from build123d import *

# Parameters (mm, degrees)
BOSS_EXTRUDE3_DEPTH       = 17
SHELL4_T                  = -2.25
SHELL4_THICKNESS_2_FACE_W = 17.75
SHELL4_THICKNESS_2_FACE_H = 12.5
SHELL4_THICKNESS_2_DEPTH  = 0.75
SHELL4_THICKNESS_3_FACE_W = 17
SHELL4_THICKNESS_3_FACE_H = 12.5
SHELL4_THICKNESS_3_DEPTH  = 0.75
CUT_EXTRUDE1_DEPTH        = 29.08914381
CUT_EXTRUDE2_DEPTH        = 29.08914381
BOSS_EXTRUDE4_DEPTH       = 1
BOSS_EXTRUDE5_DEPTH       = 1
BOSS_EXTRUDE6_DEPTH       = 1
BOSS_EXTRUDE7_DEPTH       = 1


with BuildPart() as part:
    # Sketch4 → Boss-Extrude3 (new body)
    with BuildSketch(Plane(origin=(0, 0, 0), x_dir=(0, 0, -1), z_dir=(1, 0, 0))):
        Polygon((7, 10), (-10, -7), (-10, -10), (10, -10), (10, 10), align=None)
    extrude(amount=BOSS_EXTRUDE3_DEPTH)

    # Shell4
    shell4_openings = [part.faces().sort_by_distance(p)[0] for p in [
        (8.5, 10, -8.5),
        (8.5, -8.5, 10),
        (8.5, 1.5, 1.5),
    ]]
    offset(amount=SHELL4_T, openings=shell4_openings, kind=Kind.INTERSECTION)

    # Shell4 thickness 2 face (on inner face of the shell) → Shell4 thickness 2 (add)
    with BuildSketch(Plane(origin=(8.5, -7.75, 1.125), x_dir=(0, 0, -1), z_dir=(0, -1, 0))):
        Rectangle(SHELL4_THICKNESS_2_FACE_W, SHELL4_THICKNESS_2_FACE_H)
    extrude(amount=-SHELL4_THICKNESS_2_DEPTH)

    # Shell4 thickness 3 face (on inner face of the shell) → Shell4 thickness 3 (add)
    with BuildSketch(Plane(origin=(8.5, 1.5, -7.75), x_dir=(0, -1, 0), z_dir=(0, 0, -1))):
        Rectangle(SHELL4_THICKNESS_3_FACE_W, SHELL4_THICKNESS_3_FACE_H)
    extrude(amount=-SHELL4_THICKNESS_3_DEPTH)

    # Sketch5 → Cut-Extrude1 (cut, through all)
    with BuildSketch(Plane(origin=(0, 0, -10), x_dir=(-1, 0, 0), z_dir=(0, 0, -1))):
        with BuildLine():
            Line((-11.5, 1.5), (-11.5, -1.5))
            ThreePointArc((-11.5, -1.5), (-8.5, -4.5), (-5.5, -1.5))
            Line((-5.5, -1.5), (-5.5, 1.5))
            ThreePointArc((-5.5, 1.5), (-8.5, 4.5), (-11.5, 1.5))
        make_face()
    extrude(amount=-CUT_EXTRUDE1_DEPTH, mode=Mode.SUBTRACT)

    # Sketch8 → Cut-Extrude2 (cut, through all)
    with BuildSketch(Plane(origin=(0, -10, 0), x_dir=(-1, 0, 0), z_dir=(0, -1, 0))):
        with BuildLine():
            Line((-11.5, 1.5), (-11.5, -1.5))
            ThreePointArc((-11.5, -1.5), (-8.5, -4.5), (-5.5, -1.5))
            Line((-5.5, -1.5), (-5.5, 1.5))
            ThreePointArc((-5.5, 1.5), (-8.5, 4.5), (-11.5, 1.5))
        make_face()
    extrude(amount=-CUT_EXTRUDE2_DEPTH, mode=Mode.SUBTRACT)

    # Sketch9 → Boss-Extrude4 (add)
    with BuildSketch(Plane(origin=(0, 0, -10), x_dir=(-1, 0, 0), z_dir=(0, 0, -1))):
        with BuildLine():
            Line((-9.525, 8.125), (-7.475, 8.125))
            ThreePointArc((-7.475, 8.125), (-6.6, 7.25), (-7.475, 6.375))
            Line((-7.475, 6.375), (-9.525, 6.375))
            ThreePointArc((-9.525, 6.375), (-10.4, 7.25), (-9.525, 8.125))
        make_face()
    extrude(amount=BOSS_EXTRUDE4_DEPTH)

    # Sketch10 → Boss-Extrude5 (add)
    with BuildSketch(Plane(origin=(0, 0, -10), x_dir=(-1, 0, 0), z_dir=(0, 0, -1))):
        with BuildLine():
            Line((-9.525, -6.375), (-7.475, -6.375))
            ThreePointArc((-7.475, -6.375), (-6.6, -7.25), (-7.475, -8.125))
            Line((-7.475, -8.125), (-9.525, -8.125))
            ThreePointArc((-9.525, -8.125), (-10.4, -7.25), (-9.525, -6.375))
        make_face()
    extrude(amount=BOSS_EXTRUDE5_DEPTH)

    # Sketch12 → Boss-Extrude6 (add)
    with BuildSketch(Plane(origin=(-0.843813019, -10, -7.7592784), x_dir=(-1, 0, 0), z_dir=(0, -1, 0))):
        with BuildLine():
            Line((-10.368813019, 0.3657216), (-8.318813019, 0.3657216))
            ThreePointArc((-8.318813019, 0.3657216), (-7.443813019, -0.5092784), (-8.318813019, -1.3842784))
            Line((-8.318813019, -1.3842784), (-10.368813019, -1.3842784))
            ThreePointArc((-10.368813019, -1.3842784), (-11.243813019, -0.5092784), (-10.368813019, 0.3657216))
        make_face()
    extrude(amount=BOSS_EXTRUDE6_DEPTH)

    # Sketch14 → Boss-Extrude7 (add)
    with BuildSketch(Plane(origin=(-0.843813019, -10, -7.7592784), x_dir=(-1, 0, 0), z_dir=(0, -1, 0))):
        with BuildLine():
            Line((-10.368813019, -14.1342784), (-8.318813019, -14.1342784))
            ThreePointArc((-8.318813019, -14.1342784), (-7.443813019, -15.0092784), (-8.318813019, -15.8842784))
            Line((-8.318813019, -15.8842784), (-10.368813019, -15.8842784))
            ThreePointArc((-10.368813019, -15.8842784), (-11.243813019, -15.0092784), (-10.368813019, -14.1342784))
        make_face()
    extrude(amount=BOSS_EXTRUDE7_DEPTH)


solid = part.part
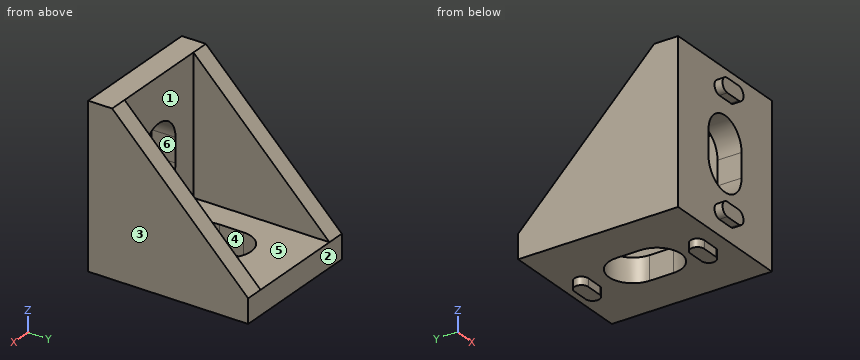
For this review, take the finished solid that the model builds, in its own axes (mm). Face numbers are marked on the shaded views. A direction names the side the tool comes from. Round coordinates to 2 decimals unless told otherwise and drop trailing zeros. Order: outer loops, then holes, each group sorted by start corner. A loop starts at its lowest first (then second) coordinate and runs counter-clockwise, first axis right, second up. Notation, with made-up numbers: M 20.5,39.25 L 56.5,39.25 A23 cw 56.5,73.25 Z; hole C -36.75,29 d4. An arc over 180 degrees is marked long. Use a Markdown table: item, result. Add a question column.
Item 1: Add section B-B, the plane y = -9.5. Give the boundary of the cut face in (x, z), then the cut area to 3 significant figures.
Item 2: To check wall thickness, follow line 1 along X through (y, z) = (-2, -3.5); line 2 along X through (y, z) = (-8, 0.25); line 3 along Z through (x, y) = (13.25, -3). State the ranges of each line that lie inside material, in increasing order.
Item 3: Add section C-C, the plane x = 8.5. State how many separate pieces and enclosed holes the cut face has, then the cut area to 3 significant figures.
Item 4: Add section A-A, the plane z = -1. Give the boundary of the cut face in (x, y), then the cut area to 3 significant figures.
Item 5: Tool access review of the marked faces 4, 5 and 6: name each direction out of +Z, -Z, +X, -X, +Y, -Y from which nothing blocks a thin tool from reaching the whole face with its end or side.
Item 6: Insertion check: pin 1 (2.5 mm diameter, centred on y = -8, z = -0.5, fed in from -X); pin 2 (10 mm diameter, centred on x = 15, z = 7, fed in from +Y); pin 3 (0.8 mm diameter, centred on x = 8, y = -10.5, fed in from -Z) (3 decimals); pin 4 (2 mm diameter, centred on x = 11, z = 0.5, fed in from +Y). Each pin has a flat end and moves straight along its axis. Give the tip position at first contact, or say it passes through.
Item 7: Add section D-D, the plane z = 7.25. Give the boundary of the cut face in (x, y).
Item 8: Mouldability with a two-part tool opening along X and no side actions: class the marked faces 1, 2 and 3 as released by +X, released by -X, zero draft, split by the parting line, or undercut.
Geometry results:
| question | item | result |
|---|---|---|
| 1 | outline | M 0,-10 L 17,-10 L 17,10 L 0,10 Z; hole M 5.5,-1.5 A3 ccw 11.5,-1.5 L 11.5,1.5 A3 ccw 5.5,1.5 Z |
| 1 | area | 294 mm² |
| 2 | line 1 | x = 0 to 2.25, 14.75 to 17 |
| 2 | line 2 | x = 0 to 5.5, 11.5 to 17 |
| 2 | line 3 | z = -10 to -7 |
| 3 | separate pieces | 3 |
| 3 | enclosed holes | 0 |
| 3 | area | 64.0 mm² |
| 4 | outline | M 0,-10 L 5.5,-10 L 5.5,-7 L 2.25,-7 L 2.25,4 L 0,4 Z; M 11.5,-10 L 17,-10 L 17,4 L 14.75,4 L 14.75,-7 L 11.5,-7 Z |
| 4 | area | 82.5 mm² |
| 5 | face 4 | +Z, -Z |
| 5 | face 5 | +Z, +Y |
| 5 | face 6 | +Y, -Y |
| 6 | pin 1 | stops at x = 0 |
| 6 | pin 2 | stops at y = 1 |
| 6 | pin 3 | stops at z = -8.125 |
| 6 | pin 4 | stops at y = -7 |
| 7 | outline | M 0,-10 L 6.6,-10 L 6.6,-11 L 10.4,-11 L 10.4,-10 L 17,-10 L 17,-4.25 L 14.75,-4.25 L 14.75,-7 L 2.25,-7 L 2.25,-4.25 L 0,-4.25 Z |
| 8 | face 1 | undercut |
| 8 | face 2 | zero draft |
| 8 | face 3 | released by +X |
